For this review, take the finished solid that the model builds, in its own axes (mm). A direction names the side the tool comes from. Give positions to 0.01 mm unless a question says otherwise; leave off trailing zeros. Loops run counter-clockwise (first coordinate to the right, second up) from the corner with the lowest first, then second, coordinate; pieces in that order, holes last.
```python
from build123d import *

# Parameters (mm, degrees)
CROQUIS1_W                   = 230
CROQUIS1_H                   = 15
SALIENTE_EXTRUIR1_DEPTH      = 2
CROQUIS2_W                   = 45
CROQUIS2_H                   = 22
SALIENTE_EXTRUIR2_DEPTH      = 5
CROQUIS3_W                   = 45
CROQUIS3_H                   = 22
SALIENTE_EXTRUIR3_DEPTH      = 5
SALIENTE_EXTRUIR4_DEPTH      = 6
SALIENTE_EXTRUIR4_DEPTH_BACK = 21
CROQUIS6_W                   = 77.325066443
CROQUIS6_H                   = 2
SALIENTE_EXTRUIR5_DEPTH      = 10
CORTAR_EXTRUIR1_REACH        = 130.721
CROQUIS9_W                   = 5
CROQUIS9_H                   = 22


with BuildPart() as part:
    # Croquis1 → Saliente-Extruir1 (new body)
    with BuildSketch(Plane(origin=(0, 0, 0), x_dir=(1, 0, 0), z_dir=(0, 1, 0))):
        with Locations((0, 4.747757848)):
            Rectangle(CROQUIS1_W, CROQUIS1_H)
    extrude(amount=SALIENTE_EXTRUIR1_DEPTH)

    # Croquis2 → Saliente-Extruir2 (add)
    with BuildSketch(Plane(origin=(115, 0, 0), x_dir=(0, 0, -1), z_dir=(1, 0, 0))):
        with Locations((4.747757848, 1)):
            Rectangle(CROQUIS2_W, CROQUIS2_H)
    extrude(amount=SALIENTE_EXTRUIR2_DEPTH)

    # Croquis3 → Saliente-Extruir3 (add)
    with BuildSketch(Plane.ZY.offset(115)):
        with Locations((-4.747757848, 1)):
            Rectangle(CROQUIS3_W, CROQUIS3_H)
    extrude(amount=SALIENTE_EXTRUIR3_DEPTH)

    # Croquis6 → Saliente-Extruir4 (add, two sides: drawn at the far end of the back side and taken through both)
    with BuildSketch(Plane(origin=(0, 0, -12.247757848), x_dir=(-1, 0, 0), z_dir=(0, 0, -1)).offset(-SALIENTE_EXTRUIR4_DEPTH_BACK)):
        with Locations((-20.080179861, 1)):
            Rectangle(CROQUIS6_W, CROQUIS6_H)
    extrude(amount=SALIENTE_EXTRUIR4_DEPTH + SALIENTE_EXTRUIR4_DEPTH_BACK)

    # Croquis7 → Saliente-Extruir5 (add)
    with BuildSketch(Plane(origin=(0, 2, 0), x_dir=(1, 0, 0), z_dir=(0, 1, 0))):
        Polygon((-18.58235336, 18.247757848), (-18.58235336, -8.752242152), (58.742713083, -8.752242152), (58.742713083, -7.252242152), (-17.08235336, -7.252242152), (-17.08235336, 16.747757848), (58.742713083, 16.747757848), (58.742713083, 18.247757848), align=None)
    extrude(amount=SALIENTE_EXTRUIR5_DEPTH)

    # Croquis9 → Cortar-Extruir1 (cut, up to next)
    with BuildSketch(Plane.XY.offset(17.752242152), mode=Mode.PRIVATE) as cortar_extruir1_sk1:
        with Locations((-117.5, 1)):
            Rectangle(CROQUIS9_W, CROQUIS9_H)
    cortar_extruir1_tool1 = extrude(cortar_extruir1_sk1.sketch, amount=-CORTAR_EXTRUIR1_REACH, mode=Mode.PRIVATE) & part.part
    # Croquis9 → Cortar-Extruir1 (cut, up to next)
    with BuildSketch(Plane.XY.offset(17.752242152), mode=Mode.PRIVATE) as cortar_extruir1_sk2:
        with Locations((117.5, 1)):
            Rectangle(CROQUIS9_W, CROQUIS9_H)
    cortar_extruir1_tool2 = extrude(cortar_extruir1_sk2.sketch, amount=-CORTAR_EXTRUIR1_REACH, mode=Mode.PRIVATE) & part.part
    add(cortar_extruir1_tool1.solids().sort_by_distance((-117.5, 1, 17.752242))[0], mode=Mode.SUBTRACT)
    add(cortar_extruir1_tool2.solids().sort_by_distance((117.5, 1, 17.752242))[0], mode=Mode.SUBTRACT)


solid = part.part
```
Q1. Consider section B-B on z = -2.5. Give the boundary of the cut face in (x, y), plus the area to 3 significant figures.
Answers:
outline: (-115, 0) - (115, 0) - (115, 2) - (-17.08, 2) - (-17.08, 12) - (-18.58, 12) - (-18.58, 2) - (-115, 2) - close
area: 475 mm2
Q2. For pin 1 Ø2 at (x, y) = (-74.5, 1.5) entering from +Z; pin 2 Ø1.5 at (x, z) = (70.5, -6) entering from +Y; pin 3 Ø0.6 at (x, y) = (91.5, 0.5) entering from -Z, all flat-tipped, find the tip position at first contact; note any pin that passes through.
Answers:
pin 1: stops at z = 2.75
pin 2: stops at y = 2
pin 3: stops at z = -12.25
Q3. Mouldability with a two-part tool opening along Z and no side actions: class faces 1 (the flat face through (20, 6, 8.752)), 2 (the flat face through (58.743, 3, 8)), 3 (the flat face through (-17.082, 7, -5)), 4 (the flat face through (20, 7, -16.748)) as +Z half, -Z half, draft (parallel to the pull), parting line (faces both ways), or undercut.
Answers:
face 1: +Z half
face 2: draft
face 3: undercut
face 4: undercut
Q4. Consider section A-A on x = 52. Give the boundary of the cut face in (y, z).
Answers:
outline: (0, -18.25) - (12, -18.25) - (12, -16.75) - (2, -16.75) - (2, 7.25) - (12, 7.25) - (12, 8.75) - (0, 8.75) - close
Q5. Consider section C-C on x = -99. Give the boundary of the cut face in (y, z).
Answers:
outline: (0, -12.25) - (2, -12.25) - (2, 2.75) - (0, 2.75) - close
Q6. Machinability: for faces 5 (the flat face through (58.743, 3, -17)), 6 (the flat face through (21, 6, -18.248)), 7 (the flat face through (-66, 2, -5)), 8 (the flat face through (21, 7, 7.252)), which of the approach directions +Z, -Z, +X, -X, +Y, -Y give a long, thin tool a straight path to every point of the face, cutting with its end or side? Answer none if there is none.
Answers:
face 5: -Z, +X, +Y, -Y
face 6: -Z, +X, -X, +Y, -Y
face 7: +Z, -Z, -X, +Y
face 8: +X, +Y
Q7. For probe 1 along Z at (x, y) = (36, 6.5); probe 2 along X at (y, z) = (5.5, -10.5); probe 3 along Y at (x, z) = (95.5, -5.75), list the stretches that pass through material, from the lowest coordinate up.
Answers:
probe 1: z = -18.25 to -16.75, 7.25 to 8.75
probe 2: x = -18.58 to -17.08
probe 3: y = 0 to 2
